Read the model definition and answer for the solid it produces. Units are mm, in the model's axes. A direction names the side the tool comes from. Round coordinates to 2 decimals unless told otherwise and drop trailing zeros. Loops run counter-clockwise (first coordinate to the right, second up) from the corner with the lowest first, then second, coordinate; pieces in that order, holes last. Notation, with made-up numbers: M 78.5,-15.75 L 83.5,-15.75 A23 cw 83.5,2.25 Z; hole C 52.5,67 d2. An arc over 180 degrees is marked long. Write each question's results on one line, items separated by ' | '.
```python
from build123d import *

# Parameters (mm, degrees)
SKETCH1_W            = 200
SKETCH1_H            = 290
BOSS_EXTRUDE2_DEPTH  = 10
BOSS_EXTRUDE4_DEPTH  = 140
SKETCH5_W            = 9
SKETCH5_H            = 9
CUT_EXTRUDE1_DEPTH   = 10
SKETCH6_R            = 3.78
CUT_EXTRUDE2_DEPTH   = 10
SKETCH7_R            = 25
CUT_EXTRUDE3_DEPTH   = 10
SKETCH8_W            = 190
SKETCH8_H            = 280
CUT_EXTRUDE4_DEPTH   = 10
SKETCH9_W            = 211.457715155
SKETCH9_H            = 301.376650104
CUT_EXTRUDE5_DEPTH   = 5
SKETCH10_W           = 200
SKETCH10_H           = 5
BOSS_EXTRUDE7_DEPTH  = 15
SKETCH12_W           = 200
SKETCH12_H           = 5
BOSS_EXTRUDE8_DEPTH  = 15
SKETCH13_W           = 290
SKETCH13_H           = 5
BOSS_EXTRUDE14_DEPTH = 190
CUT_EXTRUDE6_DEPTH   = 300
SKETCH18_W           = 9
SKETCH18_H           = 9
CUT_EXTRUDE7_DEPTH   = 10


with BuildPart() as part:
    # Sketch1 → Boss-Extrude2 (new body)
    with BuildSketch(Plane(origin=(0, 0, 0), x_dir=(1, 0, 0), z_dir=(0, 1, 0))):
        with Locations((3.938356164, -87.893835616)):
            Rectangle(SKETCH1_W, SKETCH1_H)
    extrude(amount=BOSS_EXTRUDE2_DEPTH)

    # Sketch2 → Boss-Extrude4 (add)
    with BuildSketch(Plane(origin=(0, 10, 0), x_dir=(1, 0, 0), z_dir=(0, 1, 0))):
        Polygon((-96.061643836, 57.106164384), (-96.061643836, -87.893835616), (-91.061643836, -87.893835616), (-91.061643836, 52.106164384), (3.938356164, 52.106164384), (3.938356164, 57.106164384), align=None)
        Polygon((103.938356164, 57.106164384), (3.938356164, 57.106164384), (3.938356164, 52.106164384), (98.938356164, 52.106164384), (98.938356164, -87.893835616), (103.938356164, -87.893835616), align=None)
        Polygon((3.938356164, -227.893835616), (3.938356164, -232.893835616), (103.938356164, -232.893835616), (103.938356164, -87.893835616), (98.938356164, -87.893835616), (98.938356164, -227.893835616), align=None)
        Polygon((-91.061643836, -87.893835616), (-96.061643836, -87.893835616), (-96.061643836, -232.893835616), (3.938356164, -232.893835616), (3.938356164, -227.893835616), (-91.061643836, -227.893835616), align=None)
    extrude(amount=BOSS_EXTRUDE4_DEPTH)

    # Sketch5 → Cut-Extrude1 (cut)
    with BuildSketch(Plane(origin=(103.938356164, 0, 0), x_dir=(0, 0, -1), z_dir=(1, 0, 0))):
        with Locations((-158.893835616, 143.5)):
            Rectangle(SKETCH5_W, SKETCH5_H)
        with Locations((-129.893835616, 143.5)):
            Rectangle(SKETCH5_W, SKETCH5_H)
        with Locations((-41.143835616, 143.5)):
            Rectangle(SKETCH5_W, SKETCH5_H)
    extrude(amount=-CUT_EXTRUDE1_DEPTH, mode=Mode.SUBTRACT)

    # Sketch6 → Cut-Extrude2 (cut)
    with BuildSketch(Plane.ZY.offset(96.061643836)):
        with Locations((189.256335616, 112.5)):
            Circle(SKETCH6_R)
        with Locations((-13.468664384, 112.5)):
            Circle(SKETCH6_R)
        with Locations((189.256335616, 61.57)):
            Circle(SKETCH6_R)
        with Locations((-13.468664384, 61.57)):
            Circle(SKETCH6_R)
    extrude(amount=-CUT_EXTRUDE2_DEPTH, mode=Mode.SUBTRACT)

    # Sketch7 → Cut-Extrude3 (cut)
    with BuildSketch(Plane.XY.offset(232.893835616)):
        with Locations((63.938356164, 110)):
            Circle(SKETCH7_R)
    extrude(amount=-CUT_EXTRUDE3_DEPTH, mode=Mode.SUBTRACT)

    # Sketch8 → Cut-Extrude4 (cut)
    with BuildSketch(Plane(origin=(0, 10, 0), x_dir=(1, 0, 0), z_dir=(0, 1, 0))):
        with Locations((3.938356164, -87.893835616)):
            Rectangle(SKETCH8_W, SKETCH8_H)
    extrude(amount=-CUT_EXTRUDE4_DEPTH, mode=Mode.SUBTRACT)

    # Sketch9 → Cut-Extrude5 (cut)
    with BuildSketch(Plane.XZ):
        with Locations((3.40694666, 89.005470801)):
            Rectangle(SKETCH9_W, SKETCH9_H)
    extrude(amount=-CUT_EXTRUDE5_DEPTH, mode=Mode.SUBTRACT)

    # Sketch10 → Boss-Extrude7 (add)
    with BuildSketch(Plane(origin=(0, 0, 227.893835616), x_dir=(-1, 0, 0), z_dir=(0, 0, -1))):
        with Locations((-3.938356164, 147.5)):
            Rectangle(SKETCH10_W, SKETCH10_H)
    extrude(amount=BOSS_EXTRUDE7_DEPTH)

    # Sketch12 → Boss-Extrude8 (add)
    with BuildSketch(Plane.XY.offset(-52.106164384)):
        with Locations((3.938356164, 147.5)):
            Rectangle(SKETCH12_W, SKETCH12_H)
    extrude(amount=BOSS_EXTRUDE8_DEPTH)

    # Sketch13 → Boss-Extrude14 (add)
    with BuildSketch(Plane(origin=(-91.061643836, 0, 0), x_dir=(0, 0, -1), z_dir=(1, 0, 0))):
        with Locations((-87.893835616, 132.5)):
            Rectangle(SKETCH13_W, SKETCH13_H)
    extrude(amount=BOSS_EXTRUDE14_DEPTH)

    # Sketch17 → Cut-Extrude6 (cut)
    with BuildSketch(Plane.XY.offset(232.893835616)):
        Polygon((3.938356164, 150), (-96.061643836, 150), (3.938356164, 146.51), align=None)
        Polygon((103.938356164, 150), (3.938356164, 150), (3.938356164, 146.51), align=None)
    extrude(amount=-CUT_EXTRUDE6_DEPTH, mode=Mode.SUBTRACT)

    # Sketch18 → Cut-Extrude7 (cut)
    with BuildSketch(Plane(origin=(0, 135, 0), x_dir=(1, 0, 0), z_dir=(0, 1, 0))):
        with Locations((89.633915759, -41.143835616)):
            Rectangle(SKETCH18_W, SKETCH18_H)
        with Locations((91.172972479, -129.893835616)):
            Rectangle(SKETCH18_W, SKETCH18_H)
        with Locations((91.172972479, -158.893835616)):
            Rectangle(SKETCH18_W, SKETCH18_H)
    extrude(amount=-CUT_EXTRUDE7_DEPTH, mode=Mode.SUBTRACT)


solid = part.part
```
1. Which of the six approach directions +Z, -Z, +X, -X, +Y, -Y give full straight-line access (tool end or side, diameter ignored) to faces 1 (the face through (-93.597, 109.146, 191.001)), 2 (the face through (5, 67, 227.894)), 3 (the face through (5, 140, 227.894))?
Completed:
face 1: -X | face 2: -Y | face 3: none
2. Find section C-C, the plane z = -26.5. Give the vertices of the cut face in (x, y).
Completed:
outline: M -96.06,5 L -91.06,5 L -91.06,130 L 98.94,130 L 98.94,5 L 103.94,5 L 103.94,150 L 98.94,149.83 L 98.94,135 L -91.06,135 L -91.06,149.83 L -96.06,150 Z
3. Find section B-B, the plane y = 16. Give the vertices of the cut face in (x, z), then the cut area to 3 significant figures.
Completed:
outline: M -96.06,-57.11 L 103.94,-57.11 L 103.94,232.89 L -96.06,232.89 Z; hole M -91.06,-52.11 L 98.94,-52.11 L 98.94,227.89 L -91.06,227.89 Z | area: 4,800 mm2
4. Find section D-D, the plane x = 20. Give the vertices of the cut face in (y, z).
Completed:
outline: M 5,-57.11 L 147.07,-57.11 L 147.07,-37.11 L 145,-37.11 L 145,-52.11 L 135,-52.11 L 135,227.89 L 145,227.89 L 145,212.89 L 147.07,212.89 L 147.07,232.89 L 5,232.89 L 5,227.89 L 130,227.89 L 130,-52.11 L 5,-52.11 Z
5. Given P1, Ø5.5, axis at x = 101.5, z = 161, coming from the +Y side; P2, Ø3, axis at x = -57.5, z = 20, coming from the -Y side; P3, Ø6, axis at y = 61.57, z = 189.26, coming from the -X side; P4, Ø12, axis at x = -49.5, z = -24.5, coming from the +Y side, each flat-ended and moving along its own axis, determine where each tip first touches the part or whether it passes through.
Completed:
P1: stops at y = 150 | P2: stops at y = 130 | P3: stops at x = 98.94 | P4: stops at y = 135
6. Find section A-A, the plane y = 61.57. Give the vertices of the cut face in (x, z).
Completed:
outline: M -96.06,-57.11 L 103.94,-57.11 L 103.94,232.89 L -96.06,232.89 L -96.06,193.04 L -91.06,193.04 L -91.06,227.89 L 98.94,227.89 L 98.94,-52.11 L -91.06,-52.11 L -91.06,-17.25 L -96.06,-17.25 Z; M -96.06,-9.69 L -91.06,-9.69 L -91.06,185.48 L -96.06,185.48 Z
7. Find the intervals of material crossed by L1, parallel to X at y = 95, z = 138; L2, parallel to Z at x = 36, y = 56; L3, parallel to Y at x = 9, z = 132.5, in increasing order.
Completed:
L1: x = -96.06 to -91.06, 98.94 to 103.94 | L2: z = -57.11 to -52.11, 227.89 to 232.89 | L3: y = 130 to 135
8. Determine the mould class of faces 4 (the face through (3, 67, -52.106)), 5 (the face through (5, 76, -57.106)), 6 (the face through (-96.062, 76, 86)) for opening direction Z: released by +Z, released by -Z, zero draft, split by the parting line, or undercut.
Completed:
face 4: undercut | face 5: released by -Z | face 6: zero draft
